from build123d import *

# Parameters (mm, degrees)
SKETCH1_R           = 2.2225
BOSS_EXTRUDE1_DEPTH = 2.54


with BuildPart() as part:
    # Sketch1 → Boss-Extrude1 (new body)
    with BuildSketch(Plane.XY):
        with BuildLine():
            ThreePointArc((-12.866139272, 3.133098146), (-15.8375, 0), (-12.866139272, -3.133098146))
            Line((-12.866139272, -3.133098146), (-0.20175, -3.804654641))
            ThreePointArc((-0.20175, -3.804654641), (3.81, 0), (-0.20175, 3.804654641))
            Line((-0.20175, 3.804654641), (-12.866139272, 3.133098146))
        make_face()
        with BuildLine():
            Line((-12.7, 1.55), (-6.35, 1.55))
            ThreePointArc((-6.35, 1.55), (-4.8, 0), (-6.35, -1.55))
            Line((-6.35, -1.55), (-12.7, -1.55))
            ThreePointArc((-12.7, -1.55), (-14.25, 0), (-12.7, 1.55))
        make_face(mode=Mode.SUBTRACT)
        Circle(SKETCH1_R, mode=Mode.SUBTRACT)
    extrude(amount=BOSS_EXTRUDE1_DEPTH)


solid = part.part
Could you check a few things on this model? Use its own coordinates, in mm. A direction names the side the tool comes from. Round coordinates to 2 decimals unless told otherwise and drop trailing zeros. Write each loop counter-clockwise with the first axis right and the second up, starting at its lowest first coordinate (ties: lowest second). Pieces come first, ordered by that corner, then holes. Notation, with made-up numbers: (2, 50.5) - (43, 50.5) arc R29 cw to (43, 82.5) - close; hole circle Ø1 at (83, 20). An arc over 180 degrees is marked (long way). Put each result on its own line as item: value. Start each with the question number.
(1) I want a section at C-C, the plane z = 2.35. Give the number of separate pieces and of enclosed holes in the cut face, plus the area to 3 significant figures.
(2) I want a section at D-D, the plane x = -4. Please give me the cut outline in (y, z), plus the area to 3 significant figures.
(3) Thinking about a two-plate mould opening in Y: for faces 1 (the cylindrical face through (3.81, -0.09, 1.25)), 2 (the flat face through (-10, 1.55, 1)), 3 (the flat face through (-9, -1.55, 1)), 4 (the flat face through (-4, 0, 2.54)), which applies, released by +Y, released by -Y, zero draft, split by the parting line, or undercut?
(4) I want a section at B-B, the plane y = 0. Please give me the cut outline in (x, z).
(5) I need wall thicknesses on probe 1 along Y at (x, z) = (0, 2.05); probe 2 along X at (y, z) = (-2, 0.6); probe 3 along Y at (x, z) = (-11.75, 0.75). Which ranges of each line are inside material? Lowest first, please.
(6) I want a section at A-A, the plane x = 0. Please give me the cut outline in (y, z), plus the area to 3 significant figures.
(7) For faces 5 (the cylindrical face through (-4.8, 0, 1.3)), 6 (the cylindrical face through (-15.837, 0.067, 1.252)), which set-ups out of +Z, -Z, +X, -X, +Y, -Y let a thin tool reach every point of the face, with its end or its side?
(8) Will these pins go through, and if not, where does the flat tip stop? pin 1 (1.3 mm diameter, centred on x = -10, z = 1.5, fed in from -Y); pin 2 (1 mm diameter, centred on y = 1, z = 2, fed in from -X); pin 3 (3 mm diameter, centred on x = -0.5, y = -1, fed in from -Z).
Here are the results:
1. separate pieces: 1
1. enclosed holes: 2
1. area: 83.9 mm^2
2. outline: (-3.6, 0) - (3.6, 0) - (3.6, 2.54) - (-3.6, 2.54) - close
2. area: 18.3 mm^2
3. face 1: split by the parting line
3. face 2: undercut
3. face 3: undercut
3. face 4: zero draft
4. outline: (-15.84, 0) - (-14.25, 0) - (-14.25, 2.54) - (-15.84, 2.54) - close; (-4.8, 0) - (-2.22, 0) - (-2.22, 2.54) - (-4.8, 2.54) - close; (2.22, 0) - (3.81, 0) - (3.81, 2.54) - (2.22, 2.54) - close
5. probe 1: y = -3.81 to -2.22, 2.22 to 3.81
5. probe 2: x = -15.12 to -0.97, 0.97 to 3.24
5. probe 3: y = -3.19 to -1.55, 1.55 to 3.19
6. outline: (-3.81, 0) - (-2.22, 0) - (-2.22, 2.54) - (-3.81, 2.54) - close; (2.22, 0) - (3.81, 0) - (3.81, 2.54) - (2.22, 2.54) - close
6. area: 8.06 mm^2
7. face 5: +Z, -Z
7. face 6: +Z, -Z, -X
8. pin 1: stops at y = -3.32
8. pin 2: stops at x = -15.8
8. pin 3: stops at z = 0
